from build123d import *

# Parameters (mm, degrees)
F0_W     = 10
F0_H     = 30
F1_DEPTH = 20
F2_R     = 9.99999
F3_R     = 4
F4_DEPTH = 15.001


# Not quite as in the source:
# - a fillet or chamfer is up to 0.001 mm smaller than in the source, because OpenCascade refuses the exact size


with BuildPart() as f1:
    # F0 (on Front) → F1 (new body)
    with BuildSketch(Plane.XZ):
        with Locations((0, 20)):
            Rectangle(F0_W, F0_H)
        Polygon((-5, 5), (-10, 5), (-10, 0), (10, 0), (10, 5), (5, 5), align=None)
    extrude(amount=F1_DEPTH)

    # F2 (radius 10 in the source; OpenCascade refuses exactly that, so slightly less here)
    f2_edges = [f1.edges().sort_by_distance(p)[0] for p in [
        (0, 0, 35),
        (0, -20, 35),
    ]]
    fillet(f2_edges, radius=F2_R)

    # F3 (on face) → F4 (cut, through all)
    with BuildSketch(Plane(origin=(-5, 0, 0), x_dir=(0, -1, 0), z_dir=(-1, 0, 0))):
        with Locations((10, 25)):
            Circle(F3_R)
    extrude(amount=-F4_DEPTH, mode=Mode.SUBTRACT)


solid = f1.part
Geometry: final body of the model. Coordinates: model frame, mm. A direction names the side the tool comes from. Coordinates: 2 decimals unless noted, no trailing zeros. Loops run counter-clockwise (first coordinate to the right, second up) from the corner with the lowest first, then second, coordinate; pieces in that order, holes last. Notation, with made-up numbers: (-21.75, 40.5) - (31.25, 40.5) arc R8 ccw to (31.25, 44.5) - close; hole circle Ø10 at (54.5, -39.75). An arc over 180 degrees is marked (long way). Put each result on its own line as item: value. Start each with the question number.
Q1. Cut plane B-B, the plane z = 28. Return loops of the section in (x, y), and give its area (3 significant figures).
Q2. Cut plane C-C, the plane y = -11.5. Return loops of the section in (x, z).
Q3. Pin query (flat end, axial travel): pin 1 Ø5 at (y, z) = (-10, 25) entering from -X; pin 2 Ø2 at (x, y) = (-3.5, -12) entering from +Z; pin 3 Ø12 at (y, z) = (-6.5, 29) entering from -X; pin 4 Ø6 at (y, z) = (-3.5, 25) entering from +X. Return the tip coordinate at first contact, or that it passes through.
Q4. Set-up query: faces 5 (the cylindrical face through (0.07, -3.01, 32.15)), 6 (the flat face through (-7, -10, 5)), 7 (the flat face through (5, -10, 20)). Return all of +Z, -Z, +X, -X, +Y, -Y with unobstructed straight access to the full face (end or side cutting, diameter ignored); none if empty.
Q5. Line query: line 1 (Z direction, x = 1.25, y = -10); line 2 (X direction, y = -5, z = 22); line 3 (Y direction, x = -2.25, z = 22.5). Output: solid intervals per line, ascending.
Q6. Cut plane D-D, the plane y = -4. Return loops of the section in (x, z).
Q7. Pull-direction query (Y, two-part tool) for faces 1 (the flat face through (0, 0, 10)), 2 (the cylindrical face through (0.07, -16.99, 32.15)), 3 (the flat face through (10, -10, 2)), 4 (the cylindrical face through (-0.07, -7.05, 27.7)); classes: released by +Y, released by -Y, zero draft, split by the parting line, or undercut.
Filled sheet:
1. outline: (-5, -19.54) - (5, -19.54) - (5, -12.65) - (-5, -12.65) - close; (-5, -7.35) - (5, -7.35) - (5, -0.46) - (-5, -0.46) - close
1. area: 138 mm²
2. outline: (-10, 0) - (10, 0) - (10, 5) - (5, 5) - (5, 21.29) - (-5, 21.29) - (-5, 5) - (-10, 5) - close; (-5, 28.71) - (5, 28.71) - (5, 34.89) - (-5, 34.89) - close
3. pin 1: through
3. pin 2: z = 34.95
3. pin 3: x = -5
3. pin 4: x = 5
4. face 5: +Z, +X, -X, +Y
4. face 6: +Z, -X, +Y, -Y
4. face 7: +Z, +X, +Y, -Y
5. line 1: 0 to 21, 29 to 35
5. line 2: -5 to 5
5. line 3: -20 to -13.12, -6.88 to 0
6. outline: (-10, 0) - (10, 0) - (10, 5) - (5, 5) - (5, 33) - (-5, 33) - (-5, 5) - (-10, 5) - close
7. face 1: released by +Y
7. face 2: released by -Y
7. face 3: zero draft
7. face 4: undercut
